```python
from build123d import *

# Parameters (mm, degrees)
SKETCH2_W           = 50
SKETCH2_H           = 65
SKETCH2_R           = 2
SKETCH2_R_2         = 4
BOSS_EXTRUDE1_DEPTH = 5
SKETCH3_W           = 21
SKETCH3_H           = 65
BOSS_EXTRUDE2_DEPTH = 5
SKETCH4_W           = 1
SKETCH4_H           = 65
BOSS_EXTRUDE3_DEPTH = 5
BOSS_EXTRUDE4_DEPTH = 5
SKETCH6_R           = 2
CUT_EXTRUDE1_DEPTH  = 59
SKETCH7_R           = 1.5
CUT_EXTRUDE2_DEPTH  = 10
SKETCH7_4_R         = 1.5
CUT_EXTRUDE3_DEPTH  = 10
SKETCH7_5_R         = 1.5
BOSS_EXTRUDE5_DEPTH = 5
SKETCH8_R           = 2
CUT_EXTRUDE4_DEPTH  = 10
SKETCH9_R           = 2.5
CUT_EXTRUDE5_DEPTH  = 10


with BuildPart() as part:
    # Sketch2 → Boss-Extrude1 (new body)
    with BuildSketch(Plane.XY):
        with Locations((25, 32.5)):
            Rectangle(SKETCH2_W, SKETCH2_H)
        with Locations((25, 59.5)):
            Circle(SKETCH2_R, mode=Mode.SUBTRACT)
        with Locations((13, 47.5)):
            Circle(SKETCH2_R, mode=Mode.SUBTRACT)
        with Locations((37, 47.5)):
            Circle(SKETCH2_R, mode=Mode.SUBTRACT)
        with Locations((25, 17.5)):
            Circle(SKETCH2_R_2, mode=Mode.SUBTRACT)
    extrude(amount=BOSS_EXTRUDE1_DEPTH)

    # Sketch3 → Boss-Extrude2 (add)
    with BuildSketch(Plane.XY.offset(5)):
        with Locations((-10.5, 32.5)):
            Rectangle(SKETCH3_W, SKETCH3_H)
    extrude(amount=-BOSS_EXTRUDE2_DEPTH)

    # Sketch4 → Boss-Extrude3 (add)
    with BuildSketch(Plane.XY.offset(5)):
        with Locations((-21.5, 32.5)):
            Rectangle(SKETCH4_W, SKETCH4_H)
    extrude(amount=-BOSS_EXTRUDE3_DEPTH)

    # Sketch5 → Boss-Extrude4 (add)
    with BuildSketch(Plane.XY.offset(5)):
        Polygon((-22, 17.5), (-22, 32.5), (-22, 47.5), (-28, 47.5), (-28, 17.5), align=None)
        Polygon((56, 17.5), (56, 47.5), (50, 47.5), (50, 32.5), (50, 17.5), align=None)
    extrude(amount=-BOSS_EXTRUDE4_DEPTH)

    # Sketch6 → Cut-Extrude1 (cut)
    with BuildSketch(Plane.XY.offset(5)):
        with Locations((25, 35.5)):
            Circle(SKETCH6_R)
    extrude(amount=-CUT_EXTRUDE1_DEPTH, mode=Mode.SUBTRACT)

    # Sketch7 → Cut-Extrude2 (cut)
    with BuildSketch(Plane.XY.offset(5)):
        with Locations((-17, 56.25)):
            Circle(SKETCH7_R)
        with Locations((45, 56.25)):
            Circle(SKETCH7_R)
    extrude(amount=-CUT_EXTRUDE2_DEPTH, mode=Mode.SUBTRACT)

    # Sketch7<4> → Cut-Extrude3 (cut)
    with BuildSketch(Plane.XY.offset(5)):
        with Locations((45, 8.75)):
            Circle(SKETCH7_4_R)
        with Locations((-17, 8.75)):
            Circle(SKETCH7_4_R)
    extrude(amount=-CUT_EXTRUDE3_DEPTH, mode=Mode.SUBTRACT)

    # Sketch7<5> → Boss-Extrude5 (add)
    with BuildSketch(Plane.XY.offset(5)):
        with Locations((-17, 56.25)):
            Circle(SKETCH7_5_R)
        with Locations((45, 56.25)):
            Circle(SKETCH7_5_R)
    extrude(amount=-BOSS_EXTRUDE5_DEPTH)

    # Sketch8 → Cut-Extrude4 (cut)
    with BuildSketch(Plane.XY.offset(5)):
        with Locations((-17, 8.75)):
            Circle(SKETCH8_R)
        with Locations((45, 8.75)):
            Circle(SKETCH8_R)
    extrude(amount=-CUT_EXTRUDE4_DEPTH, mode=Mode.SUBTRACT)

    # Sketch9 → Cut-Extrude5 (cut)
    with BuildSketch(Plane.XY.offset(5)):
        with Locations((25, 59.5)):
            Circle(SKETCH9_R)
        with Locations((25, 35.5)):
            Circle(SKETCH9_R)
        with Locations((13, 47.5)):
            Circle(SKETCH9_R)
        with Locations((37, 47.5)):
            Circle(SKETCH9_R)
    extrude(amount=-CUT_EXTRUDE5_DEPTH, mode=Mode.SUBTRACT)


solid = part.part
```
The model under review builds one solid part; all positions refer to its coordinate system, in mm. A direction names the side the tool comes from. Coordinates: 2 decimals unless noted, no trailing zeros. Write each loop counter-clockwise with the first axis right and the second up, starting at its lowest first coordinate (ties: lowest second). Pieces come first, ordered by that corner, then holes.
1) The part is to be moulded in two halves that separate along Y. For faces 1 (the face through (12.46, 45.06, 2.54)), 2 (the face through (13, 0, 3)), 3 (the face through (-22, 56, 3)), say which applies: pulls with the +Y half, pulls with the -Y half, needs draft (parallel to the pull), parting line crosses it, or undercut.
2) Clearance check with flat-ended pins moving along their axes: pin 1 Ø12 at (x, y) = (17.5, 58) entering from -Z; pin 2 Ø1 at (y, z) = (11.5, 3) entering from +X; pin 3 Ø1.5 at (x, z) = (-24, 3) entering from -Y; pin 4 Ø2.5 at (x, z) = (-25.5, 2) entering from +Y. State where each tip first meets the part, or that it passes through.
3) We need section A-A on x = 25. State the section outline as (y, z) points, then the cut area to 3 significant figures.
4) We need section C-C on y = 35.5. State the section outline as (x, z) points, then the cut area to 3 significant figures.
5) Machinability: for faces 4 (the face through (53, 17.5, 3)), 5 (the face through (-25, 47.5, 3)), 6 (the face through (53, 47.5, 3)), which of the approach directions +Z, -Z, +X, -X, +Y, -Y give a long, thin tool a straight path to every point of the face, cutting with its end or side? Answer none if there is none.
6) We need section D-D on z = 2.4. State the section outline as (x, y) points.
7) We need section B-B on x = 45. State the section outline as (y, z) points.
8) To check wall thickness, follow probe 1 along Y at (x, z) = (25, 2.3); probe 2 along Y at (x, z) = (45, 3.9); probe 3 along X at (y, z) = (8, 0.7). State the ranges of each line that lie inside material, in increasing order.
Answer list:
1. face 1: undercut
1. face 2: pulls with the -Y half
1. face 3: needs draft
2. pin 1: stops at z = 0
2. pin 2: stops at x = 50
2. pin 3: stops at y = 17.5
2. pin 4: stops at y = 47.5
3. outline: (0, 0) - (13.5, 0) - (13.5, 5) - (0, 5) - close; (21.5, 0) - (33, 0) - (33, 5) - (21.5, 5) - close; (38, 0) - (57, 0) - (57, 5) - (38, 5) - close; (62, 0) - (65, 0) - (65, 5) - (62, 5) - close
3. area: 235 mm2
4. outline: (-28, 0) - (22.5, 0) - (22.5, 5) - (-28, 5) - close; (27.5, 0) - (56, 0) - (56, 5) - (27.5, 5) - close
4. area: 395 mm2
5. face 4: +Z, -Z, +X, -Y
5. face 5: +Z, -Z, -X, +Y
5. face 6: +Z, -Z, +X, +Y
6. outline: (-28, 17.5) - (-22, 17.5) - (-22, 0) - (50, 0) - (50, 17.5) - (56, 17.5) - (56, 47.5) - (50, 47.5) - (50, 65) - (-22, 65) - (-22, 47.5) - (-28, 47.5) - close; hole circle Ø4 at (-17, 8.75); hole circle Ø5 at (13, 47.5); hole circle Ø8 at (25, 17.5); hole circle Ø5 at (25, 35.5); hole circle Ø5 at (25, 59.5); hole circle Ø5 at (37, 47.5); hole circle Ø4 at (45, 8.75)
7. outline: (0, 0) - (6.75, 0) - (6.75, 5) - (0, 5) - close; (10.75, 0) - (65, 0) - (65, 5) - (10.75, 5) - close
8. probe 1: y = 0 to 13.5, 21.5 to 33, 38 to 57, 62 to 65
8. probe 2: y = 0 to 6.75, 10.75 to 65
8. probe 3: x = -22 to -18.85, -15.15 to 43.15, 46.85 to 50
